from build123d import *

# Parameters (mm, degrees)
F0_W     = 3.5
F0_H     = 4.252
F1_DEPTH = 505
F2_W     = 10
F2_H     = 10
F3_DEPTH = 1


with BuildPart() as f1:
    # F0 (on Front) → F1 (new body)
    with BuildSketch(Plane.XZ):
        Polygon((1.5, 10), (-1.5, 10), (-1.5, 5.748), (-1.5, -5.748), (-1.5, -10), (1.5, -10), (1.5, -5.748), (1.5, 5.748), align=None)
        with Locations((-3.25, -7.874)):
            Rectangle(F0_W, F0_H)
        with Locations((3.25, -7.874)):
            Rectangle(F0_W, F0_H)
        with Locations((3.25, 7.874)):
            Rectangle(F0_W, F0_H)
        with Locations((-3.25, 7.874)):
            Rectangle(F0_W, F0_H)
    extrude(amount=F1_DEPTH)

    # F2 (on face) → F3 (join)
    with BuildSketch(Plane.XY.offset(10)):
        with Locations((0, -500)):
            Rectangle(F2_W, F2_H)
    extrude(amount=F3_DEPTH)


solid = f1.part
The listing builds one solid part. Answer for the finished solid, in the listing's coordinates (mm). A direction names the side the tool comes from. Give positions to 0.01 mm unless a question says otherwise; leave off trailing zeros. Order: outer loops, then holes, each group sorted by start corner. A loop starts at its lowest first (then second) coordinate and runs counter-clockwise, first axis right, second up. Notation, with made-up numbers: (37, -36) - (90, -36) arc R35 cw to (90, 1) - close; hole circle Ø10 at (-26, 15). An arc over 180 degrees is marked (long way). One line per item, written item: value. Start each with the question number.
1) A tool of negligible diameter and unlimited length cuts with its end or side. For faces 1 (the face through (1.5, -249, 0)), 2 (the face through (0, -249, -10)), 3 (the face through (0, -244, 10)), from which of +Z, -Z, +X, -X, +Y, -Y can it reach the whole face along a straight path? Write none if from no direction.
2) A cutting plane is placed at C-C on z = 1.25. Give the vertices of the cut face in (x, y), then the cut area to 4 significant figures.
3) A cutting plane is placed at B-B on y = -450.5. Give the vertices of the cut face in (x, z).
4) A cutting plane is placed at A-A on x = 3.5. Give the vertices of the cut face in (y, z), then the cut area to 3 significant figures.
5) The mould has two halves that part along Z. Classify faces 4 (the face through (-1.5, -249, 0)), 5 (the face through (0, -500, 11)), 6 (the face through (0, 0, 0)): released by +Z, released by -Z, zero draft, split by the parting line, or undercut.
6) Find the intervals of material crossed by L1, parallel to Z at x = -3.75, y = -186; L2, parallel to Z at x = 0.5, y = -275; L3, parallel to X at y = -298.5, z = 5.5, in increasing order.
7) Given pin 1 Ø3 at (y, z) = (-259, 1) entering from +X; pin 2 Ø4 at (x, y) = (3.5, -288) entering from +Z; pin 3 Ø3.5 at (y, z) = (-353, -2.5) entering from -X, each flat-ended and moving along its own axis, determine where each tip first touches the part or whether it passes through.
Answer sheet:
1. face 1: +X, +Y, -Y
1. face 2: -Z, +X, -X, +Y, -Y
1. face 3: +Z, +X, -X, +Y
2. outline: (-1.5, -505) - (1.5, -505) - (1.5, 0) - (-1.5, 0) - close
2. area: 1,515 mm2
3. outline: (-5, -10) - (5, -10) - (5, -5.75) - (1.5, -5.75) - (1.5, 5.75) - (5, 5.75) - (5, 10) - (-5, 10) - (-5, 5.75) - (-1.5, 5.75) - (-1.5, -5.75) - (-5, -5.75) - close
4. outline: (-505, -10) - (0, -10) - (0, -5.75) - (-505, -5.75) - close; (-505, 5.75) - (0, 5.75) - (0, 10) - (-495, 10) - (-495, 11) - (-505, 11) - close
4. area: 4,300 mm2
5. face 4: undercut
5. face 5: released by +Z
5. face 6: zero draft
6. L1: z = -10 to -5.75, 5.75 to 10
6. L2: z = -10 to 10
6. L3: x = -1.5 to 1.5
7. pin 1: stops at x = 1.5
7. pin 2: stops at z = 10
7. pin 3: stops at x = -1.5
